Read the model definition and answer for the solid it produces. Units are mm, in the model's axes. A direction names the side the tool comes from. Give positions to 0.01 mm unless a question says otherwise; leave off trailing zeros. Loops run counter-clockwise (first coordinate to the right, second up) from the corner with the lowest first, then second, coordinate; pieces in that order, holes last. Notation, with made-up numbers: (80, 17.25) - (100, 17.25) arc R23 cw to (100, 40.25) - close; hole circle Ø3 at (45.5, 47). An arc over 180 degrees is marked (long way). Use a Markdown table: item, result. Add a question column.
Item 1: Each of these flat-tipped pins is pushed along its axis until it touches: P1, Ø1.5, axis at y = 14.5, z = -60.5, coming from the +X side; P2, Ø4, axis at x = -76, y = 4, coming from the +Z side; P3, Ø4, axis at y = 6, z = 7.5, coming from the -X side; P4, Ø7.5, axis at x = 3, y = 12.5, coming from the +Z side. Where does it stop, or does it pass through?
Item 2: A cutting plane is placed at D-D (y = 20.25). Determine the outline of the cut face in (x, z), plus the area to 3 significant figures.
Item 3: A cutting plane is placed at B-B (y = 12). Determine the outline of the cut face in (x, z), plus the area to 3 significant figures.
Item 4: A cutting plane is placed at C-C (z = 21). Determine the outline of the cut face in (x, y), plus the area to 3 significant figures.
Item 5: Which of the six approach directions +Z, -Z, +X, -X, +Y, -Y give full straight-line access (tool end or side, diameter ignored) to faces 1 (the face through (0, 16, -58.596)), 2 (the face through (-67, 5, 10)), 3 (the face through (67, 4, 13)), 4 (the face through (79.379, 5.766, 11.479)), 5 (the face through (-67, 4, 13))?
Item 6: For a pull along X with two mould halves and no side action, classify faces 6 (the face through (-17.327, 1.788, -57.684)), 7 (the face through (86.947, -1, 4)), 8 (the face through (-0.55, 9.51, -60.08)), 9 (the face through (0, 9, -61.596)) as +X half, -X half, draft (parallel to the pull), parting line (faces both ways), or undercut.
Item 7: A cutting plane is placed at A-A (x = 0). Determine the outline of the cut face in (y, z).
Item 8: Consider probe 1 along Y at (x, z) = (0, -60); probe 2 along Z at (x, y) = (7.5, 10.5); probe 3 along Y at (x, z) = (53, -7.5). Determine where each line is inside the solid, lowest interval first. Write a range as [from, to].
from build123d import *

# Parameters (mm, degrees)
F0_W         = 30
F0_H         = 3
F1_DEPTH     = 3
F2_W         = 40
F2_H         = 13
F2_R         = 2.55
F3_DEPTH     = 3
F4_W         = 30
F4_H         = 3
F5_DEPTH     = 25
F6_R         = 2.55
F7_DEPTH     = 3
F8_T1_DEPTH  = 30
F8_T6_DEPTH  = 20.5
F8_T11_DEPTH = 20.5
F8_T17_DEPTH = 20.5
F8_T22_DEPTH = 47.5
F8_T30_DEPTH = 20.5
F8_T35_DEPTH = 47.5


# Not quite as in the source:
# - a fillet or chamfer that OpenCascade refuses, or shapes differently, is made with other operations: its cross-section is extruded or revolved along the edge and cut away or added
# - a feature names something its author has since deleted; it is built from what else it names


with BuildPart() as f1:
    # F0 (on Front) → F1 (new body)
    with BuildSketch(Plane.XZ):
        with BuildLine():
            ThreePointArc((-46.9467783772, -10), (-48, 0), (-46.9467783772, 10))
            Line((-46.9467783772, 10), (-86.9467783772, 10))
            Line((-86.9467783772, 10), (-86.9467783772, -10))
            Line((-86.9467783772, -10), (-46.9467783772, -10))
        make_face()
        with BuildLine():
            Line((86.9467783772, 10), (46.9467783772, 10))
            ThreePointArc((46.9467783772, 10), (47.7359684206, 5.0276554125), (48, 0))
            ThreePointArc((48, 0), (47.7359684206, -5.0276554125), (46.9467783772, -10))
            Line((46.9467783772, -10), (86.9467783772, -10))
            Line((86.9467783772, -10), (86.9467783772, 10))
        make_face()
        with BuildLine():
            Line((15, -58.5960524607), (15, -45.5960524607))
            ThreePointArc((15, -45.5960524607), (0, -48), (-15, -45.5960524607))
            Line((-15, -45.5960524607), (-15, -58.5960524607))
            Line((-15, -58.5960524607), (15, -58.5960524607))
        make_face()
        with BuildLine():
            ThreePointArc((-38.7298334621, 10), (0, 40), (38.7298334621, 10))
            Line((38.7298334621, 10), (46.9467783772, 10))
            ThreePointArc((46.9467783772, 10), (0, 48), (-46.9467783772, 10))
            Line((-46.9467783772, 10), (-38.7298334621, 10))
        make_face()
        with BuildLine():
            ThreePointArc((-15, -37.0809924355), (-30.0843611996, -26.3615479669), (-38.7298334621, -10))
            Line((-38.7298334621, -10), (-46.9467783772, -10))
            ThreePointArc((-46.9467783772, -10), (-35.7228298925, -32.060558705), (-15, -45.5960524607))
            Line((-15, -45.5960524607), (-15, -37.0809924355))
        make_face()
        with BuildLine():
            Line((46.9467783772, -10), (38.7298334621, -10))
            ThreePointArc((38.7298334621, -10), (30.0843611996, -26.3615479669), (15, -37.0809924355))
            Line((15, -37.0809924355), (15, -45.5960524607))
            ThreePointArc((15, -45.5960524607), (35.7228298925, -32.060558705), (46.9467783772, -10))
        make_face()
        with BuildLine():
            ThreePointArc((-38.7298334621, -10), (-40, 0), (-38.7298334621, 10))
            Line((-38.7298334621, 10), (-46.9467783772, 10))
            ThreePointArc((-46.9467783772, 10), (-48, 0), (-46.9467783772, -10))
            Line((-46.9467783772, -10), (-38.7298334621, -10))
        make_face()
        with BuildLine():
            Line((15, -45.5960524607), (15, -37.0809924355))
            ThreePointArc((15, -37.0809924355), (0, -40), (-15, -37.0809924355))
            Line((-15, -37.0809924355), (-15, -45.5960524607))
            ThreePointArc((-15, -45.5960524607), (0, -48), (15, -45.5960524607))
        make_face()
        with BuildLine():
            ThreePointArc((38.7298334621, 10), (39.6811878507, 5.0401716993), (40, 0))
            ThreePointArc((40, 0), (39.6811878507, -5.0401716993), (38.7298334621, -10))
            Line((38.7298334621, -10), (46.9467783772, -10))
            ThreePointArc((46.9467783772, -10), (47.7359684206, -5.0276554125), (48, 0))
            ThreePointArc((48, 0), (47.7359684206, 5.0276554125), (46.9467783772, 10))
            Line((46.9467783772, 10), (38.7298334621, 10))
        make_face()
        with Locations((0, -60.0960524607)):
            Rectangle(F0_W, F0_H)
        with BuildLine():
            ThreePointArc((-15, -45.5960524607), (-35.7228298925, -32.060558705), (-46.9467783772, -10))
            Line((-46.9467783772, -10), (-86.9467783772, -10))
            Line((-86.9467783772, -10), (-15, -61.5960524607))
            Line((-15, -61.5960524607), (-15, -58.5960524607))
            Line((-15, -58.5960524607), (-15, -45.5960524607))
        make_face()
        with BuildLine():
            Line((86.9467783772, -10), (46.9467783772, -10))
            ThreePointArc((46.9467783772, -10), (35.7228298925, -32.060558705), (15, -45.5960524607))
            Line((15, -45.5960524607), (15, -58.5960524607))
            Line((15, -58.5960524607), (15, -61.5960524607))
            Line((15, -61.5960524607), (86.9467783772, -10))
        make_face()
    extrude(amount=F1_DEPTH)

    # F2 (on face) → F3 (join)
    with BuildSketch(Plane.XY.offset(10)):
        with Locations((-66.9467783772, 3.5)):
            Rectangle(F2_W, F2_H)
        with Locations((-76.9467783772, 5)):
            Circle(F2_R, mode=Mode.SUBTRACT)
        with Locations((-56.9467783772, 5)):
            Circle(F2_R, mode=Mode.SUBTRACT)
        with Locations((66.9467783772, 3.5)):
            Rectangle(F2_W, F2_H)
        with Locations((56.9467783772, 5)):
            Circle(F2_R, mode=Mode.SUBTRACT)
        with Locations((76.9467783772, 5)):
            Circle(F2_R, mode=Mode.SUBTRACT)
    extrude(amount=F3_DEPTH)

    # F4 (on face) → F5 (join)
    with BuildSketch(Plane.XZ.offset(3)):
        with Locations((0, -60.0960524607)):
            Rectangle(F4_W, F4_H)
    extrude(amount=-F5_DEPTH)

    # F6 (on face) → F7 (cut, through all)
    with BuildSketch(Plane.XY.offset(-58.5960524607)):
        with Locations((0, 12)):
            Circle(F6_R)
    extrude(amount=-F7_DEPTH, mode=Mode.SUBTRACT)

    # F8: fillet of radius 7 on 3 edges, made by hand

    # F8_s2 → F8_t1 (join)
    with BuildSketch(Plane.YZ.offset(-15)):
        with BuildLine():
            ThreePointArc((0, -51.5960524607), (2.0502525317, -56.545799929), (7, -58.5960524607))
            Line((7, -58.5960524607), (0, -58.5960524607))
            Line((0, -58.5960524607), (0, -51.5960524607))
        make_face()
    extrude(amount=F8_T1_DEPTH)


with BuildPart() as f8_tool4:
    # F8_s5 → F8_t6 (new body)
    with BuildSketch(Plane.XY.offset(-58.5960524607)):
        with BuildLine():
            ThreePointArc((-15, 7), (-17.0502525317, 2.0502525317), (-22, 0))
            Line((-22, 0), (-15, 0))
            Line((-15, 0), (-15, 7))
        make_face()
    extrude(amount=-F8_T6_DEPTH)

    split(bisect_by=Plane(origin=(-34.2651759644, 0, -47.7801867313), x_dir=(0, 1, 0), z_dir=(0.5827740813, 0, 0.8126342167)), keep=Keep.TOP)


with BuildPart() as f1_1:
    add(f1.part)

    # F8_t3: union F8_tool4
    add(f8_tool4.part)


with BuildPart() as f8_tool9:
    # F8_s10 → F8_t11 (new body)
    with BuildSketch(Plane.XY.offset(-79.0960524607)):
        with BuildLine():
            ThreePointArc((15, 7), (17.0502525317, 2.0502525317), (22, 0))
            Line((22, 0), (15, 0))
            Line((15, 0), (15, 7))
        make_face()
    extrude(amount=F8_T11_DEPTH)

    split(bisect_by=Plane(origin=(34.2651759644, 0, -47.7801867313), x_dir=(0, 1, 0), z_dir=(-0.5827740813, 0, 0.8126342167)), keep=Keep.TOP)


with BuildPart() as f1_2:
    add(f1_1.part)

    # F8_t8: union F8_tool9
    add(f8_tool9.part)


with BuildPart() as f8_tool15:
    # F8_s16 → F8_t17 (new body)
    with BuildSketch(Plane.XY.offset(-61.5960524607)):
        with BuildLine():
            ThreePointArc((15, 7), (17.0502525317, 2.0502525317), (22, 0))
            Line((22, 0), (15, 0))
            Line((15, 0), (15, 7))
        make_face()
    extrude(amount=F8_T17_DEPTH)

    split(bisect_by=Plane(origin=(34.2651759644, 0, -47.7801867313), x_dir=(0, 1, 0), z_dir=(-0.5827740813, 0, 0.8126342167)), keep=Keep.TOP)

    split(bisect_by=Plane.XY.offset(-58.5960524607), keep=Keep.TOP)


with BuildPart() as f8_tool20:
    # F8_s21 → F8_t22 (new body)
    with BuildSketch(Plane.YZ.offset(32.5)):
        with BuildLine():
            ThreePointArc((0, -51.5960524607), (2.0502525317, -56.545799929), (7, -58.5960524607))
            Line((7, -58.5960524607), (0, -58.5960524607))
            Line((0, -58.5960524607), (0, -51.5960524607))
        make_face()
    extrude(amount=-F8_T22_DEPTH)

    split(bisect_by=Plane(origin=(34.2651759644, 0, -47.7801867313), x_dir=(0, 1, 0), z_dir=(-0.5827740813, 0, 0.8126342167)), keep=Keep.TOP)

    split(bisect_by=Plane.YZ.offset(15), keep=Keep.TOP)


with BuildPart() as f8_tool15_1:
    add(f8_tool15.part)

    # F8_t25: intersect F8_tool20
    add(f8_tool20.part, mode=Mode.INTERSECT)


with BuildPart() as f1_3:
    add(f1_2.part)

    # F8_t13: union F8_tool15
    add(f8_tool15_1.part)


with BuildPart() as f8_tool28:
    # F8_s29 → F8_t30 (new body)
    with BuildSketch(Plane.XY.offset(-41.0960524607)):
        with BuildLine():
            ThreePointArc((-15, 7), (-17.0502525317, 2.0502525317), (-22, 0))
            Line((-22, 0), (-15, 0))
            Line((-15, 0), (-15, 7))
        make_face()
    extrude(amount=-F8_T30_DEPTH)

    split(bisect_by=Plane(origin=(-34.2651759644, 0, -47.7801867313), x_dir=(0, 1, 0), z_dir=(0.5827740813, 0, 0.8126342167)), keep=Keep.TOP)

    split(bisect_by=Plane.XY.offset(-58.5960524607), keep=Keep.TOP)


with BuildPart() as f8_tool33:
    # F8_s34 → F8_t35 (new body)
    with BuildSketch(Plane.YZ.offset(15)):
        with BuildLine():
            ThreePointArc((0, -51.5960524607), (2.0502525317, -56.545799929), (7, -58.5960524607))
            Line((7, -58.5960524607), (0, -58.5960524607))
            Line((0, -58.5960524607), (0, -51.5960524607))
        make_face()
    extrude(amount=-F8_T35_DEPTH)

    split(bisect_by=Plane(origin=(-34.2651759644, 0, -47.7801867313), x_dir=(0, 1, 0), z_dir=(0.5827740813, 0, 0.8126342167)), keep=Keep.TOP)

    split(bisect_by=Plane.YZ.offset(-15), keep=Keep.BOTTOM)


with BuildPart() as f8_tool28_1:
    add(f8_tool28.part)

    # F8_t38: intersect F8_tool33
    add(f8_tool33.part, mode=Mode.INTERSECT)


with BuildPart() as f1_4:
    add(f1_3.part)

    # F8_t26: union F8_tool28
    add(f8_tool28_1.part)


solid = f1_4.part
Geometry says:
| question | item | result |
|---|---|---|
| 1 | P1 | x = 15 |
| 1 | P2 | z = 13 |
| 1 | P3 | through |
| 1 | P4 | z = -58.6 |
| 2 | outline | (-15, -61.6) - (15, -61.6) - (15, -58.6) - (-15, -58.6) - close |
| 2 | area | 90.0 mm² |
| 3 | outline | (-15, -61.6) - (-2.55, -61.6) - (-2.55, -58.6) - (-15, -58.6) - close; (2.55, -61.6) - (15, -61.6) - (15, -58.6) - (2.55, -58.6) - close |
| 3 | area | 74.7 mm² |
| 4 | outline | (-43.16, -3) - (-34.04, -3) - (-34.04, 0) - (-43.16, 0) - close; (34.04, -3) - (43.16, -3) - (43.16, 0) - (34.04, 0) - close |
| 4 | area | 54.7 mm² |
| 5 | face 1 | +Z, +X, -X, +Y |
| 5 | face 2 | -Z, +X, -X, +Y |
| 5 | face 3 | +Z, +X, +Y, -Y |
| 5 | face 4 | +Z, -Z |
| 5 | face 5 | +Z, -X, +Y, -Y |
| 6 | face 6 | -X half |
| 6 | face 7 | +X half |
| 6 | face 8 | undercut |
| 6 | face 9 | draft |
| 7 | outline | (-3, -61.6) - (9.45, -61.6) - (9.45, -58.6) - (7, -58.6) arc R7 cw to (0, -51.6) - (0, -40) - (-3, -40) - close; (-3, 40) - (0, 40) - (0, 48) - (-3, 48) - close; (14.55, -61.6) - (22, -61.6) - (22, -58.6) - (14.55, -58.6) - close |
| 8 | probe 1 | [-3, 9.45], [14.55, 22] |
| 8 | probe 2 | [-61.6, -58.6] |
| 8 | probe 3 | [-3, 0] |
